The drawing under review shows one solid part. Ordinate dimensions are in mm from its lowest x, y, z. A direction names the side the tool comes from. Coordinates: 2 decimals unless noted, no trailing zeros. Order: outer loops, then holes, each group sorted by start corner. A loop starts at its lowest first (then second) coordinate and runs counter-clockwise, first axis right, second up. Notation, with made-up numbers: (-1.75, 86) -> (20.25, 86) arc R20 ccw to (20.25, 111) -> close; hole circle Ø4 at (19.5, -15). An arc over 180 degrees is marked (long way). Put each result on its own line as item: value.
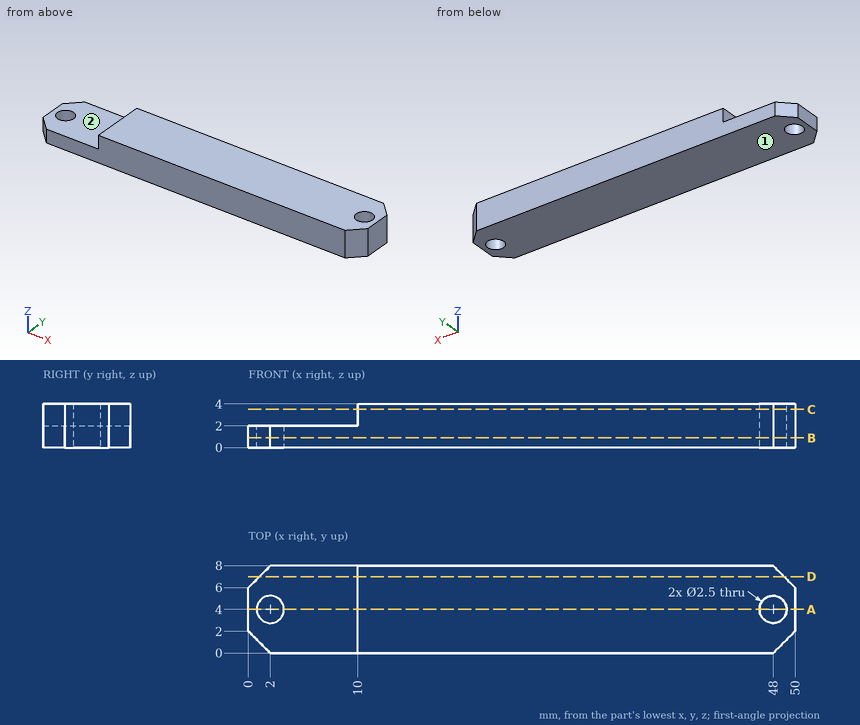
Item 1: For the marked faces 1 and 2, list the 3-axis set-ups (+Z, -Z, +X, -X, +Y, -Y) from which the entire face can be reached by the end or side of a thin tool; tool diameter is ignored.
Answers below:
face 1: -Z, +X, -X, +Y, -Y
face 2: +Z, -X, +Y, -Y
Item 2: For line 1 (X direction, y = 4, z = 2.3); line 2 (X direction, y = 5, z = 1.05); line 3 (Y direction, x = 48, z = 3.25), list the stretches that pass through material, from the lowest coordinate up. Write a range as from..to.
Answers below:
line 1: 10..46.75, 49.25..50
line 2: 0..1.25, 2.75..47.25, 48.75..50
line 3: 0..2.75, 5.25..8
Item 3: For pin 1 Ø2 at (x, y) = (48, 4) entering from -Z; pin 2 Ø1 at (y, z) = (4.5, 3.5) entering from -X, all flat-tipped, find the tip position at first contact; note any pin that passes through.
Answers below:
pin 1: through
pin 2: x = 10
Item 4: Consider section B-B on z = 0.9. Write out the cut boundary in (x, y).
Answers below:
outline: (0, 2) -> (2, 0) -> (48, 0) -> (50, 2) -> (50, 6) -> (48, 8) -> (2, 8) -> (0, 6) -> close; hole circle Ø2.5 at (2, 4); hole circle Ø2.5 at (48, 4)
Item 5: Consider section D-D on y = 7. Write out the cut boundary in (x, z).
Answers below:
outline: (1, 0) -> (49, 0) -> (49, 4) -> (10, 4) -> (10, 2) -> (1, 2) -> close
Item 6: Consider section C-C on z = 3.5. Write out the cut boundary in (x, y), and give its area (3 significant figures).
Answers below:
outline: (10, 0) -> (48, 0) -> (50, 2) -> (50, 6) -> (48, 8) -> (10, 8) -> close; hole circle Ø2.5 at (48, 4)
area: 311 mm^2
Item 7: Consider section A-A on y = 4. Write out the cut boundary in (x, z), and give its area (3 significant figures).
Answers below:
outline: (0, 0) -> (0.75, 0) -> (0.75, 2) -> (0, 2) -> close; (3.25, 0) -> (46.75, 0) -> (46.75, 4) -> (10, 4) -> (10, 2) -> (3.25, 2) -> close; (49.25, 0) -> (50, 0) -> (50, 4) -> (49.25, 4) -> close
area: 165 mm^2
